Geometry: final body of the model. Coordinates: model frame, mm. Round coordinates to 2 decimals unless told otherwise and drop trailing zeros. Write each loop counter-clockwise with the first axis right and the second up, starting at its lowest first coordinate (ties: lowest second). Pieces come first, ordered by that corner, then holes.
Autodesk Inventor part; units mm, degrees
ref_plane "YZ Plane" through (0, 0, 0) normal (1, 0, 0) x (0, 1, 0)
ref_plane "XZ Plane" through (0, 0, 0) normal (0, 1, 0) x (-1, 0, 0)
ref_plane "XY Plane" through (0, 0, 0) normal (0, 0, 1) x (1, 0, 0)
sketch "Sketch1" plane through (0, 0, 0) normal (0, 0, 1) x (1, 0, 0)
  line L0 (0, 0) -> (609.6, 0) construction
  line L1 (609.6, 0) -> (609.6, 209.55)
  line L2 (609.6, 209.55) -> (0, 209.55) construction
  line L3 (0, 209.55) -> (0, 0) construction
  line L4 (0, 0) -> (304.8, 0) construction
  line L5 (304.8, 0) -> (304.8, 165.1) construction
  line L6 (304.8, 165.1) -> (0, 165.1) construction
  line L7 (0, 165.1) -> (0, 0) construction
  line L8 (0, 0) -> (165.1, 0) construction
  line L9 (165.1, 0) -> (165.1, 304.8) construction
  line L10 (165.1, 304.8) -> (0, 304.8) construction
  line L11 (0, 304.8) -> (0, 0) construction
  line L12 (0, 0) -> (177.8, 0) construction
  line L13 (177.8, 0) -> (177.8, 177.8) construction
  line L14 (177.8, 177.8) -> (0, 177.8) construction
  line L15 (0, 177.8) -> (0, 0) construction
  circle A0 centre (177.8, 177.8) radius 12.7
  line L16 (177.8, 177.8) -> (165.1, 177.8)
  line L17 (177.8, 177.8) -> (177.8, 165.1)
  line L18 (177.8, 177.8) -> (168.819744, 168.819744)
  line L19 (177.8, 177.8) -> (190.5, 177.8) construction
  line L20 (168.819744, 168.819744) -> (52.076414, 52.076414) construction
  line L21 (168.819744, 168.819744) -> (333.919744, 168.819744) construction
  line L22 (177.8, 165.1) -> (177.8, 0) construction
  line L23 (165.1, 177.8) -> (0, 177.8) construction
  arc A1 (0, 177.8) -> (177.8, 0) centre (177.8, 177.8) ccw
  line L24 (177.8, 177.8) -> (304.8, 177.8) construction
  line L25 (304.8, 177.8) -> (304.8, 193.675)
  line L26 (304.8, 193.675) -> (177.8, 193.675) construction
  line L27 (177.8, 193.675) -> (177.8, 177.8) construction
  circle A2 centre (304.8, 193.675) radius 12.7
  line L28 (304.8, 193.675) -> (431.8, 193.675) construction
  line L29 (431.8, 193.675) -> (431.8, 209.55) construction
  line L30 (431.8, 209.55) -> (304.8, 209.55) construction
  line L31 (304.8, 209.55) -> (304.8, 193.675) construction
  circle A3 centre (431.8, 209.55) radius 12.7
  line L32 (177.8, 0) -> (609.6, 0)
  line L33 (177.8, 165.1) -> (304.8, 180.975)
  line L34 (431.8, 196.85) -> (304.8, 180.975)
  line L35 (431.8, 196.85) -> (609.6, 209.55)
  line L36 (165.1, 177.8) -> (165.1, 304.8) construction
  line L37 (165.1, 304.8) -> (241.3, 304.8) construction
  circle A4 centre (241.3, 304.8) radius 76.2
  circle A5 centre (177.8, 228.6) radius 12.7
  line L38 (177.8, 177.8) -> (177.8, 228.6)
  line L39 (0, 177.8) -> (0, 304.8)
  line L40 (241.3, 304.8) -> (195.441695, 365.656026) construction
  line L41 (241.3, 304.8) -> (317.5, 304.8) construction
  line L42 (195.441695, 365.656026) -> (354.191695, 365.656026) construction
  line L43 (195.441695, 365.656026) -> (99.90356, 492.439413) construction
  line L44 (195.441695, 365.656026) -> (354.191695, 365.656026) construction
  line L45 (165.1, 304.8) -> (0, 304.8) construction
  line L46 (241.3, 304.8) -> (169.695422, 330.861935) construction
  line L47 (241.3, 304.8) -> (317.5, 304.8) construction
  line L48 (169.695422, 330.861935) -> (20.519219, 385.157633) construction
  line L49 (177.8, 0) -> (408.09644, 0) construction
  line L50 (241.3, 304.8) -> (317.5, 304.8) construction
  line L51 (241.3, 304.8) -> (175.308864, 342.9) construction
  line L52 (241.3, 304.8) -> (317.5, 304.8) construction
  line L53 (175.308864, 342.9) -> (37.827331, 422.275) construction
  arc A6 (99.90356, 492.439413) -> (20.519219, 385.157633) centre (241.3, 304.8) ccw
  arc A7 (37.827331, 422.275) -> (0, 304.8) centre (330.4977, 263.206429) ccw
  line L54 (37.827331, 422.275) -> (26.828809, 428.625) construction
  circle A8 centre (26.828809, 428.625) radius 12.7
  line L55 (0, 304.8) -> (-12.7, 304.8) construction
  circle A9 centre (-12.7, 304.8) radius 12.7
  line L56 (0, 177.8) -> (-12.7, 177.8) construction
  circle A10 centre (-12.7, 177.8) radius 12.7
  line L57 (52.076414, 52.076414) -> (43.096158, 43.096158) construction
  circle A11 centre (43.096158, 43.096158) radius 12.7
  line L58 (0, 177.8) -> (0, 304.8)
  circle A12 centre (43.096158, 43.096158) radius 11.1125
  circle A13 centre (-12.7, 304.8) radius 11.1125
  circle A14 centre (-12.7, 177.8) radius 11.1125
  circle A15 centre (26.828809, 428.625) radius 11.1125
  line L59 (190.5, 177.8) -> (393.7, 177.8) construction
  line L60 (609.6, 0) -> (-50.8, 0)
  line L61 (-50.8, 0) -> (-50.8, 508)
  line L62 (-50.8, 508) -> (99.90356, 492.439413)
  line L63 (177.8, 0) -> (-50.8, 0)
  point P0 (165.275068, 230.701449)
  point P1 (172.715134, 216.962383)
  dimension "d16" = 25.4
  dimension "d19" = 25.4
  dimension "d0" = 609.6
  dimension "d1" = 209.55
  dimension "d2" = 304.8
  dimension "d3" = 165.1
  dimension "d4" = 165.1
  dimension "d5" = 304.8
  dimension "d6" = 177.8
  dimension "d7" = 177.8
  dimension "d8" = 25.4
  dimension "d9" = 12.7
  dimension "d10" = 135
  dimension "d11" = 165.1
  dimension "d12" = 135
  dimension "d13" = 165.1
  dimension "d14" = 127
  dimension "d15" = 15.875
  dimension "d17" = 127
  dimension "d18" = 15.875
  dimension "d20" = 127
  dimension "d21" = 76.2
  dimension "d22" = 152.4
  dimension "d23" = 25.4
  dimension "d24" = 50.8
  dimension "d25" = 127
  dimension "d26" = 127
  dimension "d33" = 158.75
  dimension "d34" = 127
  dimension "d35" = 160
  dimension "d36" = 158.75
  dimension "d37" = 180
  dimension "d45" = 150
  dimension "d46" = 158.75
  dimension "d47" = 180
  dimension "d48" = 12.7
  dimension "d49" = 12.7
  dimension "d50" = 12.7
  dimension "d52" = 12.7
  dimension "d53" = 25.4
  dimension "d55" = 214.47119
  dimension "d56" = 22.225
  dimension "d57" = 22.225
  dimension "d58" = 22.225
  dimension "d59" = 22.225
  dimension "d60" = 134.70384
  dimension "d72" = 660.4
  dimension "d73" = 508
  dimension "d74" = 90
sketch "Sketch1 outline for Extrusion2" plane through (0, 0, 0) normal (0, 0, 1) x (1, 0, 0)
  line L0 (-50.8, 508) -> (-50.8, 0)
  line L1 (99.90356, 492.439413) -> (-50.8, 508)
  line L2 (-50.8, 0) -> (177.8, 0)
  arc A0 (37.827331, 422.275) -> (99.90356, 492.439413) centre (241.3, 304.8) cw
  arc A1 (177.8, 0) -> (0, 177.8) centre (177.8, 177.8) cw
  arc A2 (20.519219, 385.157633) -> (37.827331, 422.275) centre (241.3, 304.8) cw
  line L3 (0, 177.8) -> (0, 304.8)
  arc A3 (0, 304.8) -> (20.519219, 385.157633) centre (330.4977, 263.206429) cw
  circle A4 centre (-12.7, 177.8) radius 11.1125
  circle A5 centre (43.096158, 43.096158) radius 11.1125
  circle A6 centre (-12.7, 304.8) radius 11.1125
  circle A7 centre (26.828809, 428.625) radius 11.1125
extrude "Extrusion2" add sketch "Sketch1 outline for Extrusion2" along normal blind 25.4
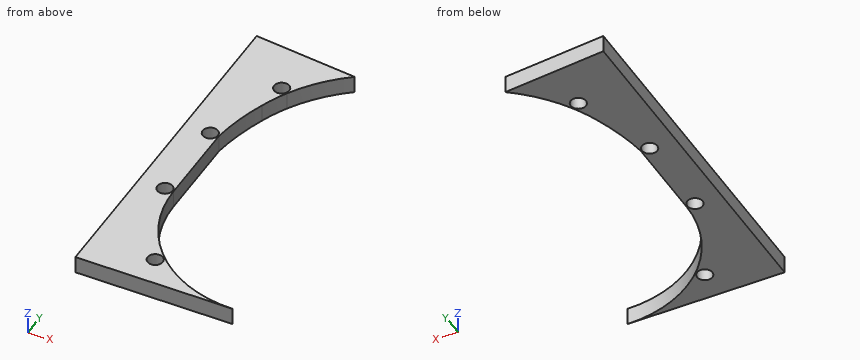
1) Section D-D on y = 471.5. Output: boundary loops of the cut face in (x, z), plus the area to 3 significant figures.
2) First-contact query: P1, Ø10, axis at y = 274.5, z = 8, coming from the +X side; P2, Ø6, axis at y = 150.5, z = 3.5, coming from the +X side; P3, Ø10, axis at x = -26.5, z = 11, coming from the +Y side; P4, Ø20, axis at x = 26.83, y = 428.62, coming from the -Z side. Flat tips, straight axial feed; report the tip coordinate or a pass-through.
3) Section A-A on x = -12.7. Output: boundary loops of the cut face in (y, z).
4) Section C-C on x = 83. Output: boundary loops of the cut face in (y, z), plus the area to 3 significant figures.
5) Line query: probe 1 along Y at (x, z) = (25, 3.5); probe 2 along Y at (x, z) = (26.5, 15.75); probe 3 along Y at (x, z) = (88, 15). Output: solid intervals per line, ascending.
6) Section B-B on z = 19.75. State how many separate pieces and enclosed holes the cut face has, plus the area to 3 significant figures.
Filled in:
1. outline: (-50.8, 0) - (75.73, 0) - (75.73, 25.4) - (-50.8, 25.4) - close
1. area: 3,210 mm2
2. P1: stops at x = 0
2. P2: stops at x = 2.6
2. P3: stops at y = 506.01
2. P4: passes through
3. outline: (0, 0) - (166.69, 0) - (166.69, 25.4) - (0, 25.4) - close; (188.91, 0) - (293.69, 0) - (293.69, 25.4) - (188.91, 25.4) - close; (315.91, 0) - (504.07, 0) - (504.07, 25.4) - (315.91, 25.4) - close
4. outline: (0, 0) - (27.38, 0) - (27.38, 25.4) - (0, 25.4) - close; (478.42, 0) - (494.18, 0) - (494.18, 25.4) - (478.42, 25.4) - close
4. area: 1,100 mm2
5. probe 1: y = 0 to 86.89, 396.54 to 417.66, 439.59 to 500.17
5. probe 2: y = 0 to 84.41, 400 to 417.52, 439.73 to 500.02
5. probe 3: y = 0 to 24.34, 482.85 to 493.67
6. separate pieces: 1
6. enclosed holes: 4
6. area: 37,700 mm2
